Verification items for the finished model (mm, model axes). Face numbers are marked on the shaded views. A direction names the side the tool comes from. Give positions to 0.01 mm unless a question says otherwise; leave off trailing zeros. Order: outer loops, then holes, each group sorted by start corner. A loop starts at its lowest first (then second) coordinate and runs counter-clockwise, first axis right, second up. Notation, with made-up numbers: (29.5, 39) -> (39.5, 39) arc R19 cw to (39.5, 64) -> close; hole circle Ø8 at (13.5, -11). An arc over 180 degrees is marked (long way). Return JSON: item names as keys, results as strings. Group by question number.
(1) Thickness scan on line 1 along Y through (x, z) = (22.5, 2.8); line 2 along Y through (x, z) = (0, 5.5); line 3 along Y through (x, z) = (0, 1.5). Record the ranges inside material, lowest first.
(2) Release check for a two-part mould opening along X. For the marked faces 1 and 2 record: pulls with the +X half, pulls with the -X half, needs draft (parallel to the pull), parting line crosses it, or undercut.
(3) Depth check by flat-ended pin: pin 1 Ø4 at (x, y) = (0, 0) entering from +Z; pin 2 Ø5 at (x, y) = (22.5, -22.5) entering from +Z. Enter the tip coordinate at first touch or a pass-through.
(4) Cross-section at A-A on x = -22.5. Enter the section's corners in (y, z).
(5) Cross-section at B-B on y = 0. Enter the section's corners in (x, z), then the cut area to 3 significant figures.
(6) Tool access check on the marked faces 3 and 4. Record the directions out of +Z, -Z, +X, -X, +Y, -Y that give a thin tool (end or side, any length) a straight path to the whole face; none if there is none.
from build123d import *

# Parameters (mm, degrees)
SKETCH1_W           = 55
SKETCH1_H           = 55
SKETCH1_R           = 3.2
SKETCH1_R_2         = 2
BOSS_EXTRUDE1_DEPTH = 5
SKETCH2_R           = 18.2
SKETCH2_R_2         = 3.2
BOSS_EXTRUDE2_DEPTH = 2


with BuildPart() as part:
    # Sketch1 → Boss-Extrude1 (new body)
    with BuildSketch(Plane.XY):
        Rectangle(SKETCH1_W, SKETCH1_H)
        Circle(SKETCH1_R, mode=Mode.SUBTRACT)
        with Locations((-22.5, 22.5)):
            Circle(SKETCH1_R_2, mode=Mode.SUBTRACT)
        with Locations((22.5, 22.5)):
            Circle(SKETCH1_R_2, mode=Mode.SUBTRACT)
        with Locations((-22.5, -22.5)):
            Circle(SKETCH1_R_2, mode=Mode.SUBTRACT)
        with Locations((22.5, -22.5)):
            Circle(SKETCH1_R_2, mode=Mode.SUBTRACT)
    extrude(amount=BOSS_EXTRUDE1_DEPTH)

    # Sketch2 → Boss-Extrude2 (add)
    with BuildSketch(Plane.XY.offset(5)):
        Circle(SKETCH2_R)
        Circle(SKETCH2_R_2, mode=Mode.SUBTRACT)
    extrude(amount=BOSS_EXTRUDE2_DEPTH)


solid = part.part
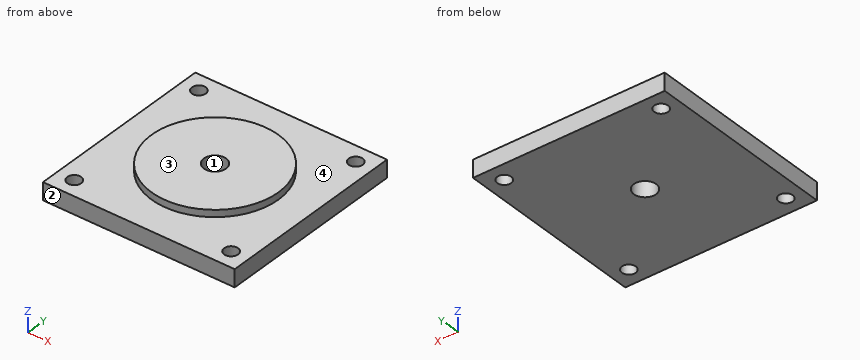
Verdict:
{
 "1": {"line 1": "-27.5 to -24.5, -20.5 to 20.5, 24.5 to 27.5", "line 2": "-18.2 to -3.2, 3.2 to 18.2", "line 3": "-27.5 to -3.2, 3.2 to 27.5"},
 "2": {"face 1": "undercut", "face 2": "needs draft"},
 "3": {"pin 1": "through", "pin 2": "z = 5"},
 "4": {"outline": "(-27.5, 0) -> (-24.5, 0) -> (-24.5, 5) -> (-27.5, 5) -> close; (-20.5, 0) -> (20.5, 0) -> (20.5, 5) -> (-20.5, 5) -> close; (24.5, 0) -> (27.5, 0) -> (27.5, 5) -> (24.5, 5) -> close"},
 "5": {"outline": "(-27.5, 0) -> (-3.2, 0) -> (-3.2, 7) -> (-18.2, 7) -> (-18.2, 5) -> (-27.5, 5) -> close; (3.2, 0) -> (27.5, 0) -> (27.5, 5) -> (18.2, 5) -> (18.2, 7) -> (3.2, 7) -> close", "area": "303 mm²"},
 "6": {"face 3": "+Z, +X, -X, +Y, -Y", "face 4": "+Z"}
}
